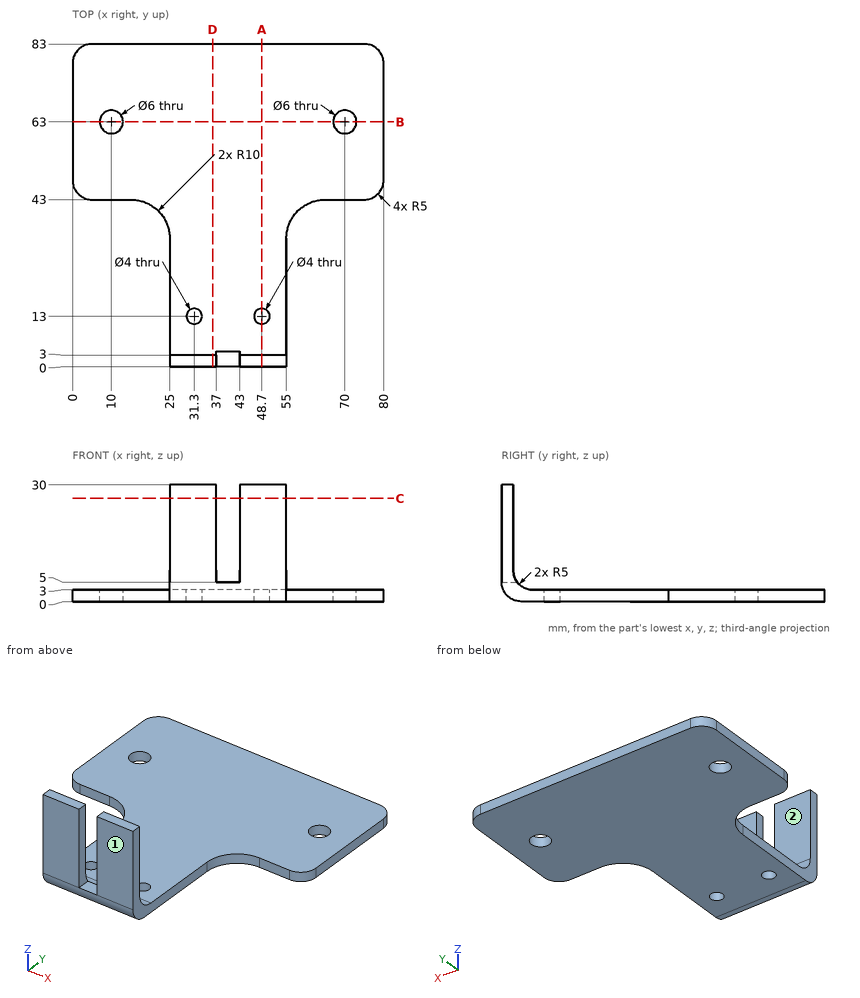
Input: dimensioned drawing with shaded views. Units: mm. Origin: part minimum x, y, z. A direction names the side the tool comes from. Round coordinates to 2 decimals unless told otherwise and drop trailing zeros. Order: outer loops, then holes, each group sorted by start corner. A loop starts at its lowest first (then second) coordinate and runs counter-clockwise, first axis right, second up. Notation, with made-up numbers: (-28, 77.5) -> (2, 77.5) arc R29 cw to (2, 98.5) -> close; hole circle Ø9 at (1.25, 21). An arc over 180 degrees is marked (long way). Put each result on its own line as item: value. Start each with the question number.
Q1. Line query: probe 1 along X at (y, z) = (63, 1.8); probe 2 along X at (y, z) = (13, 2.4); probe 3 along Y at (x, z) = (70, 2.15). Output: solid intervals per line, ascending.
Q2. Section D-D on x = 36. Return the cut outline in (y, z), and give its area (3 significant figures).
Q3. Reachability of the marked faces 1 and 2 from +Z, -Z, +X, -X, +Y, -Y: full face, straight path, thin tool, end or side. Return the list, or none.
Q4. Section A-A on x = 48.7. Return the cut outline in (y, z), and give its area (3 significant figures).
Q5. Section B-B on y = 63. Return the cut outline in (x, z).
Q6. Section C-C on z = 26.5. Return the cut outline in (x, y), and give its area (3 significant figures).
Q7. First-contact query: pin 1 (1.2 mm diameter, centred on x = 41, y = 2, fed in from +Z); pin 2 (6 mm diameter, centred on x = 42.5, y = 42.5, fed in from +Z); pin 3 (5 mm diameter, centred on x = 36.5, z = 25.5, fed in from +Y). Flat tips, straight axial feed; report the tip coordinate or a pass-through.
Ans:
1. probe 1: x = 0 to 7, 13 to 67, 73 to 80
1. probe 2: x = 25 to 29.3, 33.3 to 46.7, 50.7 to 55
1. probe 3: y = 43 to 60, 66 to 83
2. outline: (0, 5) arc R5 ccw to (5, 0) -> (83, 0) -> (83, 3) -> (8, 3) arc R5 cw to (3, 8) -> (3, 30) -> (0, 30) -> close
2. area: 330 mm2
3. face 1: +Z, -Z, +X, -X, -Y
3. face 2: +Z, +X, -X, +Y
4. outline: (0, 5) arc R5 ccw to (5, 0) -> (11, 0) -> (11, 3) -> (8, 3) arc R5 cw to (3, 8) -> (3, 30) -> (0, 30) -> close; (15, 0) -> (83, 0) -> (83, 3) -> (15, 3) -> close
4. area: 318 mm2
5. outline: (0, 0) -> (7, 0) -> (7, 3) -> (0, 3) -> close; (13, 0) -> (67, 0) -> (67, 3) -> (13, 3) -> close; (73, 0) -> (80, 0) -> (80, 3) -> (73, 3) -> close
6. outline: (25, 0) -> (37, 0) -> (37, 3) -> (25, 3) -> close; (43, 0) -> (55, 0) -> (55, 3) -> (43, 3) -> close
6. area: 72.0 mm2
7. pin 1: stops at z = 5
7. pin 2: stops at z = 3
7. pin 3: stops at y = 3
